from build123d import *

# Parameters (mm, degrees)
CROQUIS1_R              = 12
CROQUIS1_R_2            = 2.5
SALIENTE_EXTRUIR1_DEPTH = 4
CORTAR_EXTRUIR1_DEPTH   = 4


with BuildPart() as part:
    # Croquis1 → Saliente-Extruir1 (new body)
    with BuildSketch(Plane(origin=(0, 0, 0), x_dir=(1, 0, 0), z_dir=(0, 1, 0))):
        with Locations(Location((0, 0, 0), (0, 0, 270))):
            Circle(CROQUIS1_R)
        with Locations(Location((0, 0, 0), (0, 0, 270))):
            Circle(CROQUIS1_R_2, mode=Mode.SUBTRACT)
    extrude(amount=SALIENTE_EXTRUIR1_DEPTH)

    # Croquis3 → Cortar-Extruir1 (cut)
    with BuildSketch(Plane(origin=(0, 4, 0), x_dir=(1, 0, 0), z_dir=(0, 1, 0))):
        Polygon((15.178438839, 8.150766492), (6.84734968, 2.265789565), (4.424123887, 5.696238042), (12.755213045, 11.581214969), align=None)
        Polygon((-4.424123887, -5.696238042), (-6.84734968, -2.265789565), (-15.178438839, -8.150766492), (-12.755213045, -11.581214969), align=None)
        Polygon((12.755213045, -11.581214969), (4.424123887, -5.696238042), (6.84734968, -2.265789565), (15.178438839, -8.150766492), align=None)
        Polygon((-6.84734968, 2.265789565), (-4.424123887, 5.696238042), (-12.755213045, 11.581214969), (-15.178438839, 8.150766492), align=None)
    extrude(amount=-CORTAR_EXTRUIR1_DEPTH, mode=Mode.SUBTRACT)


solid = part.part
Model file for the job. Use its own axes, mm. A direction names the side the tool comes from. Coordinates: 2 decimals unless noted, no trailing zeros. Loops run counter-clockwise (first coordinate to the right, second up) from the corner with the lowest first, then second, coordinate; pieces in that order, holes last. Notation, with made-up numbers: (59, -23.75) -> (71, -23.75) arc R23 ccw to (71, -14.75) -> close; hole circle Ø8 at (-14.75, 40.25). An arc over 180 degrees is marked (long way). Use one line per item in the form item = value. Start each with the question number.
(1) Pull direction Z, two halves, no side cores. Call faces 1 (the flat face through (6.459, 2.028, 7.134)), 2 (the cylindrical face through (12, 2, 0)), 3 (the flat face through (3, 0, 0)): pulls with the +Z half, pulls with the -Z half, needs draft (parallel to the pull), parting line crosses it, or undercut.
(2) Cut at A-A on z = 0. Give the cut face in (x, y).
(3) Flat gauge pin, fed straight in: pin 1 (2 mm diameter, centred on y = 2.5, z = -5, fed in from +X). Where does the tip first touch, or does it go through?
(4) Probe probe 1 along X at (y, z) = (1.8, 4); probe 2 along Z at (x, y) = (-7.25, 0.45); probe 3 along Z at (x, y) = (5.75, 3.05). List the from-to ranges inside material, lowest first. Write a range as from..to.
(5) Cut at D-D on x = -5.25. Give the cut face in (y, z).
(6) Cut at C-C on x = 0. Give the cut face in (y, z).
(7) Tool access for faces 4 (the flat face through (-8.88, 2.03, -3.7)), 5 (the flat face through (-6.459, 2.028, 7.134)), 6 (the flat face through (3, 4, 0)): list every direction of +Z, -Z, +X, -X, +Y, -Y with a clear straight run to the whole face (end or side of a thin tool).
(8) Cut at B-B on y = 0.7. Give the cut face in (x, z), and give its area (3 significant figures).
Values:
q1.face_1 = undercut
q1.face_2 = parting line crosses it
q1.face_3 = needs draft
q2.outline = (-12, 0) -> (-2.5, 0) -> (-2.5, 4) -> (-12, 4) -> close; (2.5, 0) -> (12, 0) -> (12, 4) -> (2.5, 4) -> close
q3.pin_1 = 11.31
q4.probe_1 = -11.31..-9.3, -5.62..5.62, 9.3..11.31
q4.probe_2 = -9.56..-7.69, -2.55..2.55, 7.69..9.56
q4.probe_3 = -10.53..-6.63, -3.82..3.82, 6.63..10.53
q5.outline = (0, -10.79) -> (4, -10.79) -> (4, -6.28) -> (0, -6.28) -> close; (0, -4.53) -> (4, -4.53) -> (4, 4.53) -> (0, 4.53) -> close; (0, 6.28) -> (4, 6.28) -> (4, 10.79) -> (0, 10.79) -> close
q6.outline = (0, -12) -> (4, -12) -> (4, -2.5) -> (0, -2.5) -> close; (0, 2.5) -> (4, 2.5) -> (4, 12) -> (0, 12) -> close
q7.face_4 = +Y, -Y
q7.face_5 = -X, +Y, -Y
q7.face_6 = +Z, -Z, +X, -X, +Y
q8.outline = (-10.86, -5.1) -> (-6.85, -2.27) -> (-4.42, -5.7) -> (-8.44, -8.53) arc R12 ccw to (8.44, -8.53) -> (4.42, -5.7) -> (6.85, -2.27) -> (10.86, -5.1) arc R12 ccw to (10.86, 5.1) -> (6.85, 2.27) -> (4.42, 5.7) -> (8.44, 8.53) arc R12 ccw to (-8.44, 8.53) -> (-4.42, 5.7) -> (-6.85, 2.27) -> (-10.86, 5.1) arc R12 ccw to start; hole circle Ø5 at (0, 0)
q8.area = 348 mm2
